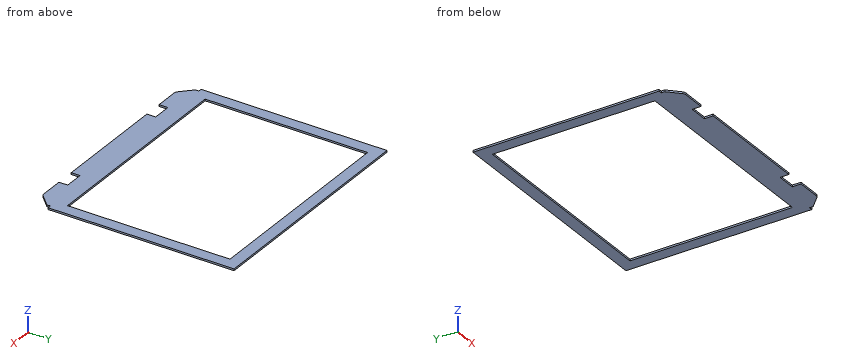
```python
from build123d import *

# Parameters (mm, degrees)
SKETCH1_W           = 400
SKETCH1_H           = 317
SKETCH1_W_2         = 360
SKETCH1_H_2         = 277
BOSS_EXTRUDE1_DEPTH = 3
BOSS_EXTRUDE4_DEPTH = 3


with BuildPart() as part:
    # Sketch1 → Boss-Extrude1 (new body)
    with BuildSketch(Plane.XY):
        Rectangle(SKETCH1_W, SKETCH1_H)
        Rectangle(SKETCH1_W_2, SKETCH1_H_2, mode=Mode.SUBTRACT)
    extrude(amount=BOSS_EXTRUDE1_DEPTH)

    # Sketch2 → Boss-Extrude4 (add, through all)
    with BuildSketch(Plane.XY.offset(3)):
        with BuildLine():
            Line((-98.955345629, -185), (0, -185))
            Line((0, -185), (0, -158.5))
            Line((0, -158.5), (-194, -158.5))
            Line((-194, -158.5), (-194, -164.5))
            Line((-194, -164.5), (-175.383585865, -183.116414135))
            ThreePointArc((-175.383585865, -183.116414135), (-173.093720589, -184.544378238), (-170.433838397, -185))
            Line((-170.433838397, -185), (-130.955345629, -185))
            Line((-130.955345629, -185), (-130.955345629, -170))
            Line((-130.955345629, -170), (-98.955345629, -170))
            Line((-98.955345629, -170), (-98.955345629, -185))
        make_face()
        with BuildLine():
            Line((130.955345629, -170), (130.955345629, -185))
            Line((130.955345629, -185), (170.433838397, -185))
            ThreePointArc((170.433838397, -185), (173.093720589, -184.544378238), (175.383585865, -183.116414135))
            Line((175.383585865, -183.116414135), (194, -164.5))
            Line((194, -164.5), (194, -158.5))
            Line((194, -158.5), (0, -158.5))
            Line((0, -158.5), (0, -185))
            Line((0, -185), (98.955345629, -185))
            Line((98.955345629, -185), (98.955345629, -170))
            Line((98.955345629, -170), (130.955345629, -170))
        make_face()
    extrude(amount=-BOSS_EXTRUDE4_DEPTH)


solid = part.part
```
Input: part model. Units: mm. Frame: model coordinates. Give positions to 0.01 mm unless a question says otherwise; leave off trailing zeros. Order: outer loops, then holes, each group sorted by start corner. A loop starts at its lowest first (then second) coordinate and runs counter-clockwise, first axis right, second up. Notation, with made-up numbers: (39.5, 69) - (56.5, 69) arc R30 cw to (56.5, 96) - close; hole circle Ø1 at (11, 26). An arc over 180 degrees is marked (long way). Use a Markdown table: item, result.
(1) Line query: line 1 (X direction, y = 71.5, z = 2.35); line 2 (Y direction, x = 32, z = 0.25); line 3 (Y direction, x = -110.5, z = 2.1). Output: solid intervals per line, ascending. Write a range as from..to.
Computed values:
| item | result |
|---|---|
| line 1 | x = -200..-180, 180..200 |
| line 2 | y = -185..-138.5, 138.5..158.5 |
| line 3 | y = -170..-138.5, 138.5..158.5 |
(2) Section query B-B (y = 32.5). Output: boundary loops of the cut face in (x, z), then the cut area to 3 significant figures.
Computed values:
| item | result |
|---|---|
| outline | (-200, 0) - (-180, 0) - (-180, 3) - (-200, 3) - close; (180, 0) - (200, 0) - (200, 3) - (180, 3) - close |
| area | 120 mm2 |
(3) Section query A-A (x = 138). Output: boundary loops of the cut face in (y, z).
Computed values:
| item | result |
|---|---|
| outline | (-185, 0) - (-138.5, 0) - (-138.5, 3) - (-185, 3) - close; (138.5, 0) - (158.5, 0) - (158.5, 3) - (138.5, 3) - close |
(4) Pin query (flat end, axial travel): pin 1 (1.5 mm diameter, centred on x = -197.5, z = 2, fed in from -Y); pin 2 (1.5 mm diameter, centred on y = -163, z = 1, fed in from +X); pin 3 (1.5 mm diameter, centred on x = 122.5, z = 1.5, fed in from -Y). Return the tip coordinate at first contact, or that it passes through.
Computed values:
| item | result |
|---|---|
| pin 1 | stops at y = -158.5 |
| pin 2 | stops at x = 194 |
| pin 3 | stops at y = -170 |
(5) Section query C-C (z = 1.7). Output: boundary loops of the cut face in (x, y), then the cut area to 3 significant figures.
Computed values:
| item | result |
|---|---|
| outline | (-200, -158.5) - (-194, -158.5) - (-194, -164.5) - (-175.38, -183.12) arc R7 ccw to (-170.43, -185) - (-130.96, -185) - (-130.96, -170) - (-98.96, -170) - (-98.96, -185) - (98.96, -185) - (98.96, -170) - (130.96, -170) - (130.96, -185) - (170.43, -185) arc R7 ccw to (175.38, -183.12) - (194, -164.5) - (194, -158.5) - (200, -158.5) - (200, 158.5) - (-200, 158.5) - close; hole (-180, -138.5) - (180, -138.5) - (180, 138.5) - (-180, 138.5) - close |
| area | 36,000 mm2 |
